from build123d import *

# Parameters (mm, degrees)
SKETCH1_W           = 40
SKETCH1_H           = 16
BOSS_EXTRUDE1_DEPTH = 2
SKETCH2_W           = 40
SKETCH2_H           = 16
SKETCH2_W_2         = 38
SKETCH2_H_2         = 14
BOSS_EXTRUDE2_DEPTH = 2
BOSS_EXTRUDE5_REACH = 45.267
SKETCH3_R           = 2.75
SKETCH4_R           = 1.75
CUT_EXTRUDE1_DEPTH  = 44.266615306


with BuildPart() as part:
    # Sketch1 → Boss-Extrude1 (new body)
    with BuildSketch(Plane(origin=(0, 0, 0), x_dir=(1, 0, 0), z_dir=(0, 1, 0))):
        with Locations((20, 8)):
            Rectangle(SKETCH1_W, SKETCH1_H)
    extrude(amount=BOSS_EXTRUDE1_DEPTH)

    # Sketch2 → Boss-Extrude2 (add)
    with BuildSketch(Plane(origin=(0, 2, 0), x_dir=(1, 0, 0), z_dir=(0, 1, 0))):
        with Locations((20, 8)):
            Rectangle(SKETCH2_W, SKETCH2_H)
        with Locations((20, 8)):
            Rectangle(SKETCH2_W_2, SKETCH2_H_2, mode=Mode.SUBTRACT)
    extrude(amount=BOSS_EXTRUDE2_DEPTH)

    # Sketch3 → Boss-Extrude5 (add, up to next)
    with BuildSketch(Plane(origin=(0, 4, 0), x_dir=(1, 0, 0), z_dir=(0, 1, 0)), mode=Mode.PRIVATE) as boss_extrude5_sk1:
        with Locations((17.75, 13.25)):
            Circle(SKETCH3_R)
    boss_extrude5_tool1 = extrude(boss_extrude5_sk1.sketch, amount=-BOSS_EXTRUDE5_REACH, mode=Mode.PRIVATE) - part.part
    # Sketch3 → Boss-Extrude5 (add, up to next)
    with BuildSketch(Plane(origin=(0, 4, 0), x_dir=(1, 0, 0), z_dir=(0, 1, 0)), mode=Mode.PRIVATE) as boss_extrude5_sk2:
        with Locations((36.75, 13.25)):
            Circle(SKETCH3_R)
    boss_extrude5_tool2 = extrude(boss_extrude5_sk2.sketch, amount=-BOSS_EXTRUDE5_REACH, mode=Mode.PRIVATE) - part.part
    add(boss_extrude5_tool1.solids().sort_by_distance((17.75, 4, -13.25))[0])
    add(boss_extrude5_tool2.solids().sort_by_distance((36.75, 4, -13.25))[0])

    # Sketch4 → Cut-Extrude1 (cut, through all)
    with BuildSketch(Plane(origin=(0, 4, 0), x_dir=(1, 0, 0), z_dir=(0, 1, 0))):
        with Locations(Location((17.75, 13.25, 0), (0, 0, 270))):
            Circle(SKETCH4_R)
        with Locations(Location((36.75, 13.25, 0), (0, 0, 270))):
            Circle(SKETCH4_R)
    extrude(amount=-CUT_EXTRUDE1_DEPTH, mode=Mode.SUBTRACT)


solid = part.part
Could you check a few things on this model? Use its own coordinates, in mm. A direction names the side the tool comes from. Give positions to 0.01 mm unless a question says otherwise; leave off trailing zeros. Write each loop counter-clockwise with the first axis right and the second up, starting at its lowest first coordinate (ties: lowest second). Pieces come first, ordered by that corner, then holes. Notation, with made-up numbers: (80.5, 21.25) -> (107.5, 21.25) arc R24 cw to (107.5, 53.25) -> close; hole circle Ø4 at (-32.5, -11.75). An arc over 180 degrees is marked (long way). Answer as CSV lines item,"result". Start each with the question number.
(1) If we mould it in two halves opening along X, with no side actions, what happens to faces 3 (the face through (35.04, 2.03, -13.63)), 4 (the face through (40, 2, -8)), 5 (the face through (20, 4, -12))? For each: +X half, -X half, draft (parallel to the pull), parting line (faces both ways), or undercut.
(2) If we section it at D-D, the plane y = 0.5: Write out the boundary of the cut face in (x, z), and give its area (3 significant figures).
(3) If we section it at C-C, the plane x = 17.75: Write out the boundary of the cut face in (y, z), and give its area (3 significant figures).
(4) Please list where these lines run through material, in increasing order: line 1 (X direction, y = 2.4, z = -13.25); line 2 (X direction, y = 1.45, z = -13.25); line 3 (Z direction, x = 28, y = 3.6).
(5) I'm going to push a flat-ended pin straight in: pin 1 Ø2 at (x, y) = (23, 0.5) entering from +Z. Where does the tip first touch, or does it pass through?
(6) If we section it at B-B, the plane z = -13.25: Write out the boundary of the cut face in (x, y).
(7) If we section it at A-A, the plane y = 3.3: Write out the boundary of the cut face in (x, z).
(8) Which directions (+Z, -Z, +X, -X, +Y, -Y) give clear straight access to the entire face, cutting with the end or side of a thin tool? Please do faces 1 (the face through (20, 3, -1)), 2 (the face through (20, 2, -16)).
Answer list:
1,face 3,"undercut"
1,face 4,"+X half"
1,face 5,"draft"
2,outline,"(0, -16) -> (40, -16) -> (40, 0) -> (0, 0) -> close; hole circle Ø3.5 at (17.75, -13.25); hole circle Ø3.5 at (36.75, -13.25)"
2,area,"621 mm^2"
3,outline,"(0, -16) -> (4, -16) -> (4, -15) -> (0, -15) -> close; (0, -11.5) -> (4, -11.5) -> (4, -10.5) -> (2, -10.5) -> (2, -1) -> (4, -1) -> (4, 0) -> (0, 0) -> close"
3,area,"31.0 mm^2"
4,line 1,"0 to 1, 15 to 16, 19.5 to 20.5, 34 to 35, 38.5 to 40"
4,line 2,"0 to 16, 19.5 to 35, 38.5 to 40"
4,line 3,"-16 to -15, -1 to 0"
5,pin 1,"z = 0"
6,outline,"(0, 0) -> (16, 0) -> (16, 4) -> (15, 4) -> (15, 2) -> (1, 2) -> (1, 4) -> (0, 4) -> close; (19.5, 0) -> (35, 0) -> (35, 4) -> (34, 4) -> (34, 2) -> (20.5, 2) -> (20.5, 4) -> (19.5, 4) -> close; (38.5, 0) -> (40, 0) -> (40, 4) -> (38.5, 4) -> close"
7,outline,"(0, -16) -> (40, -16) -> (40, 0) -> (0, 0) -> close; hole (1, -15) -> (15.63, -15) arc R2.75 cw (long way) to (19.87, -15) -> (34.63, -15) arc R2.75 cw (long way) to (39, -11.67) -> (39, -1) -> (1, -1) -> close; hole circle Ø3.5 at (17.75, -13.25); hole circle Ø3.5 at (36.75, -13.25); hole (38.87, -15) -> (39, -15) -> (39, -14.83) arc R2.75 cw to start"
8,face 1,"+Y"
8,face 2,"-Z, +X, -X, +Y, -Y"
